from build123d import *

# Parameters (mm, degrees)
FILLET_1_R             = 2
CHAMFER_1_SIZE         = 1.5
CHAMFER_1_SIZE2        = 2.598076211
HOLE_WIZARD_M5_1_D     = 4.2
HOLE_WIZARD_M5_1_DEPTH = 12.4
HOLE_WIZARD_M5_1_TIP   = 1.2618073


with BuildPart() as part:
    # 草图1 → 旋转1 (revolve)
    with BuildSketch(Plane.XY, mode=Mode.PRIVATE) as revolve_1_sk:
        with BuildLine():
            Line((0, 13), (0, 18))
            Line((0, 18), (-12, 18))
            Line((-12, 18), (-12, 16))
            Line((-12, 16), (-31, 16))
            ThreePointArc((-31, 16), (-42.313708499, 11.313708499), (-47, 0))
            Line((-47, 0), (-43, 0))
            ThreePointArc((-43, 0), (-39.485281374, 8.485281374), (-31, 12))
            Line((-31, 12), (-15, 12))
            Line((-15, 12), (-15, 13))
            Line((-15, 13), (0, 13))
        make_face()
    revolve(revolve_1_sk.sketch.rotate(Axis((-47, 0, 0), (1, 0, 0)), 90), axis=Axis((-47, 0, 0), (1, 0, 0)))

    # 圆角1
    fillet_1_edges = [part.edges().sort_by_distance(p)[0] for p in [
        (-12, 0, -16),
    ]]
    fillet(fillet_1_edges, radius=FILLET_1_R - 0.0001)  # a hair under: the kernel refuses the full size

    # 倒角1
    chamfer_1_edges = [part.edges().sort_by_distance(p)[0] for p in [
        (0, 0, -13),
    ]]
    chamfer_1_side = [part.faces().sort_by_distance(p)[0] for p in [
        (-7.5, 0, -13),
    ]]
    chamfer(chamfer_1_edges, length=CHAMFER_1_SIZE, length2=CHAMFER_1_SIZE2, reference=chamfer_1_side[0])

    # M5 螺纹孔1
    with Locations(Plane(origin=(-6, 18, 0), x_dir=(0, 0, 1), z_dir=(0, 1, 0))):
        with Locations((0, 0)):
            Hole(HOLE_WIZARD_M5_1_D / 2, depth=HOLE_WIZARD_M5_1_DEPTH)
            with Locations((0, 0, -(HOLE_WIZARD_M5_1_DEPTH + HOLE_WIZARD_M5_1_TIP / 2))):  # 118° drill point
                Cone(0, HOLE_WIZARD_M5_1_D / 2, HOLE_WIZARD_M5_1_TIP, mode=Mode.SUBTRACT)


solid = part.part
Model file for the job. Use its own axes, mm. A direction names the side the tool comes from. Round coordinates to 2 decimals unless told otherwise and drop trailing zeros. Order: outer loops, then holes, each group sorted by start corner. A loop starts at its lowest first (then second) coordinate and runs counter-clockwise, first axis right, second up.
(1) Pin check, flat tips, straight feed: pin 1 (19 mm diameter, centred on y = 0, z = 0, fed in from +X); pin 2 (8 mm diameter, centred on y = 0, z = 9.5, fed in from +X); pin 3 (6 mm diameter, centred on y = -13, z = 1.5, fed in from -X). Stop position of each tip, or through.
(2) Drill centre lines: line 1 (Y direction, x = -27.25, z = 0); line 2 (Z direction, x = -42, y = -1); line 3 (Y direction, x = -18.5, z = -5.5). Where is each one in solid material? Low to high.
(3) 3-axis set-ups, long thin cutter, end or side, ignore diameter. For faces 1 (the face through (-8.156, 7.91, -10.316)), 2 (the face through (-22.62, 15.62, -3.47)), 3 (the face through (0, -15, 5)): which of +Z, -Z, +X, -X, +Y, -Y reach the whole face in a straight line?
(4) Band-saw the part on B-B (x = -37). List the corners of the cut face in (y, z).
(5) Pull direction X, two halves, no side cores. Call faces 4 (the face through (-1.41, -3.95, 12.55)), 5 (the face through (-8.05, 15.38, 0.46)), 6 (the face through (-22.888, -3.604, 11.446)): released by +X, released by -X, zero draft, split by the parting line, or undercut.
(6) Band-saw the part on C-C (x = -10.5). List the corners of the cut face in (y, z), then the cut area to 3 significant figures.
Verdict:
1. pin 1: stops at x = -38.33
1. pin 2: stops at x = -1.21
1. pin 3: stops at x = -43.42
2. line 1: y = -16 to -12, 12 to 16
2. line 2: z = -11.58 to -4.69, 4.69 to 11.58
2. line 3: y = -15.02 to -10.67, 10.67 to 15.02
3. face 1: +X
3. face 2: -X
3. face 3: +Z, -Z, +X, +Y, -Y
4. outline: circle Ø29.66 at (0, 0); hole circle Ø20.78 at (0, 0)
5. face 4: released by +X
5. face 5: undercut
5. face 6: zero draft
6. outline: circle Ø36 at (0, 0); hole circle Ø26 at (0, 0)
6. area: 487 mm2
